```python
from build123d import *

# Parameters (mm, degrees)
SKETCH1_W               = 60
SKETCH1_H               = 60
SKETCH1_W_2             = 54
SKETCH1_H_2             = 54
BOSS_EXTRUDE1_DEPTH     = 180
FILLET1_R               = 3
SKETCH2_R               = 6
CUT_EXTRUDE1_DEPTH      = 31
CUT_EXTRUDE1_DEPTH_BACK = 31


with BuildPart() as part:
    # Sketch1 → Boss-Extrude1 (new body)
    with BuildSketch(Plane.XY):
        Rectangle(SKETCH1_W, SKETCH1_H)
        Rectangle(SKETCH1_W_2, SKETCH1_H_2, mode=Mode.SUBTRACT)
    extrude(amount=BOSS_EXTRUDE1_DEPTH)

    # Fillet1
    fillet1_edges = [part.edges().sort_by_distance(p)[0] for p in [
        (27, -27, 90),
        (27, 27, 90),
        (-27, 27, 90),
        (-27, -27, 90),
        (30, -30, 90),
        (-30, -30, 90),
        (-30, 30, 90),
        (30, 30, 90),
    ]]
    fillet(fillet1_edges, radius=FILLET1_R)

    # Sketch2 → Cut-Extrude1 (cut, two sides)
    with BuildSketch(Plane(origin=(0, 0, 0), x_dir=(1, 0, 0), z_dir=(0, 1, 0))) as cut_extrude1_sk:
        with Locations((0, -90)):
            Circle(SKETCH2_R)
    extrude(amount=CUT_EXTRUDE1_DEPTH, mode=Mode.SUBTRACT)
    extrude(cut_extrude1_sk.sketch, amount=-CUT_EXTRUDE1_DEPTH_BACK, mode=Mode.SUBTRACT)


solid = part.part
```
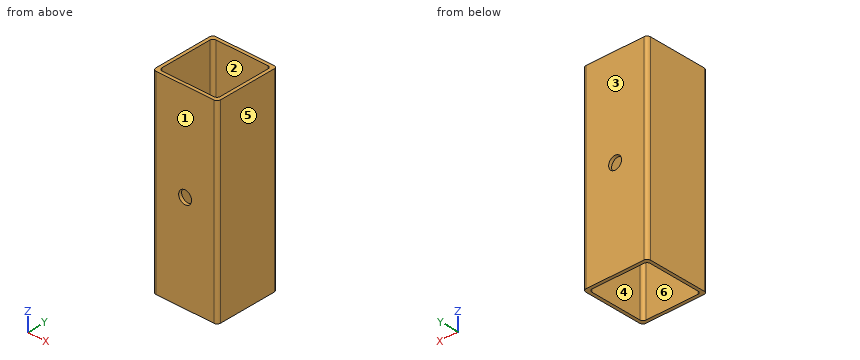
Geometry check sheet. Reference: the model listing, model coordinates, mm. Face numbers are marked on the shaded views. A direction names the side the tool comes from. Coordinates: 2 decimals unless noted, no trailing zeros. Order: outer loops, then holes, each group sorted by start corner. A loop starts at its lowest first (then second) coordinate and runs counter-clockwise, first axis right, second up. Notation, with made-up numbers: (46.5, -4.5) - (69.5, -4.5) arc R7 ccw to (69.5, -0.5) - close; hole circle Ø8 at (73.5, 64). An arc over 180 degrees is marked (long way). Answer as a JSON object with one key per item and string values. Group by question number.
Item 1: Scan lines: probe 1 along X at (y, z) = (8, 134.5); probe 2 along Z at (x, y) = (0, -28). Record each from-to range of solid material in increasing order.
Item 2: Depth check by flat-ended pin: pin 1 Ø11 at (x, z) = (0, 90) entering from -Y. Enter the tip coordinate at first touch or a pass-through.
Item 3: Tool access check on the marked faces 1 and 2. Record the directions out of +Z, -Z, +X, -X, +Y, -Y that give a thin tool (end or side, any length) a straight path to the whole face; none if there is none.
Item 4: Draft check along Y on the marked faces 3, 4, 5 and 6. Enter one of: +Y half, -Y half, draft (parallel to the pull), parting line (faces both ways), or undercut.
Item 5: Sectioned sample at B-B, the plane x = 0. Record the cut outline in (y, z).
Item 6: Sectioned sample at C-C, the plane y = -7. Record the cut outline in (x, z), and give its area (3 significant figures).
Item 7: Sectioned sample at A-A, the plane z = 90. Record the cut outline in (x, y).
Resolved:
{
 "1": {"probe 1": "-30 to -27, 27 to 30", "probe 2": "0 to 84, 96 to 180"},
 "2": {"pin 1": "through"},
 "3": {"face 1": "+Z, -Z, +X, -X, -Y", "face 2": "+Z, -Z"},
 "4": {"face 3": "+Y half", "face 4": "undercut", "face 5": "draft", "face 6": "undercut"},
 "5": {"outline": "(-30, 0) - (-27, 0) - (-27, 84) - (-30, 84) - close; (-30, 96) - (-27, 96) - (-27, 180) - (-30, 180) - close; (27, 0) - (30, 0) - (30, 84) - (27, 84) - close; (27, 96) - (30, 96) - (30, 180) - (27, 180) - close"},
 "6": {"outline": "(-30, 0) - (-27, 0) - (-27, 180) - (-30, 180) - close; (27, 0) - (30, 0) - (30, 180) - (27, 180) - close", "area": "1,080 mm^2"},
 "7": {"outline": "(-30, -27) arc R3 ccw to (-27, -30) - (-6, -30) - (-6, -27) - (-24, -27) arc R3 cw to (-27, -24) - (-27, 24) arc R3 cw to (-24, 27) - (-6, 27) - (-6, 30) - (-27, 30) arc R3 ccw to (-30, 27) - close; (6, -30) - (27, -30) arc R3 ccw to (30, -27) - (30, 27) arc R3 ccw to (27, 30) - (6, 30) - (6, 27) - (24, 27) arc R3 cw to (27, 24) - (27, -24) arc R3 cw to (24, -27) - (6, -27) - close"}
}
